from build123d import *

# Parameters (mm, degrees)
SKETCH5_R           = 14
SKETCH5_R_2         = 4
BOSS_EXTRUDE3_DEPTH = 12.5
BOSS_EXTRUDE4_DEPTH = 5


with BuildPart() as part:
    # Sketch5 → Boss-Extrude3 (new body)
    with BuildSketch(Plane(origin=(0, 0, 0), x_dir=(1, 0, 0), z_dir=(0, 1, 0))):
        with Locations(Location((0, 0, 0), (0, 0, 270))):
            Circle(SKETCH5_R)
        with Locations(Location((0, 0, 0), (0, 0, 270))):
            Circle(SKETCH5_R_2, mode=Mode.SUBTRACT)
    extrude(amount=BOSS_EXTRUDE3_DEPTH)

    # Sketch6 → Boss-Extrude4 (add)
    with BuildSketch(Plane(origin=(0, 12.5, 0), x_dir=(1, 0, 0), z_dir=(0, 1, 0))):
        with BuildLine():
            ThreePointArc((0, 14), (-12.934313455, -5.357568053), (9.899494937, -9.899494937))
            ThreePointArc((9.899494937, -9.899494937), (9.899494937, -7.071067812), (7.071067812, -7.071067812))
            ThreePointArc((7.071067812, -7.071067812), (-9.238795325, -3.826834324), (0, 10))
            ThreePointArc((0, 10), (2, 12), (0, 14))
        make_face()
    extrude(amount=BOSS_EXTRUDE4_DEPTH)


solid = part.part
Design review of the part built by this model. Coordinates are the model's own, in mm. A direction names the side the tool comes from. Give positions to 0.01 mm unless a question says otherwise; leave off trailing zeros. Write each loop counter-clockwise with the first axis right and the second up, starting at its lowest first coordinate (ties: lowest second). Pieces come first, ordered by that corner, then holes. Notation, with made-up numbers: M 16.25,-4 L 72.25,-4 A23 ccw 72.25,26 Z; hole C -21,68.5 d9. An arc over 180 degrees is marked long. Return JSON: item names as keys, results as strings. Group by question number.
Item 1: Take a section at B-B (x = -3). Give the boundary of the cut face in (y, z).
Item 2: Tool access review of faces 5 (the flat face through (-3, 0, 3)), 6 (the cylindrical face through (9.93, 14.96, 7.1)): name each direction out of +Z, -Z, +X, -X, +Y, -Y from which nothing blocks a thin tool from reaching the whole face with its end or side.
Item 3: Take a section at C-C (y = 6.5). Give the boundary of the cut face in (x, z), plus the area to 3 significant figures.
Item 4: Wall thickness on line 1 along X through (y, z) = (4.5, 0); line 2 along Y through (x, z) = (7.5, -9); line 3 along X through (y, z) = (13.85, 0): over which ranges is each line inside the solid? List them lowest first.
Item 5: The part is to be moulded in two halves that separate along X. For faces 1 (the cylindrical face through (-9.13, 14.96, 4.08)), 2 (the flat face through (-9, 17.5, 5)), 3 (the cylindrical face through (2, 15, -12)), 4 (the cylindrical face through (-3.905, 6.162, -0.867)), say which applies: pulls with the +X half, pulls with the -X half, needs draft (parallel to the pull), parting line crosses it, or undercut.
Item 6: Take a section at A-A (z = 0). Give the boundary of the cut face in (x, y), plus the area to 3 significant figures.
Item 7: Clearance check with flat-ended pins moving along their axes: pin 1 Ø12 at (x, z) = (0.5, -3) entering from +Y; pin 2 Ø3 at (x, y) = (-4.5, 6.5) entering from -Z; pin 3 Ø1 at (x, y) = (10, 14.5) entering from +Z. State where each tip first meets the part, or that it passes through.
Item 8: Take a section at D-D (z = -6.25). Give the boundary of the cut face in (x, y).
Return value:
{
 "1": {"outline": "M 0,-13.67 L 17.5,-13.67 L 17.5,-9.54 L 12.5,-9.54 L 12.5,-2.65 L 0,-2.65 Z; M 0,2.65 L 12.5,2.65 L 12.5,9.54 L 17.5,9.54 L 17.5,13.67 L 0,13.67 Z"},
 "2": {"face 5": "+Z, -Z, +X, -X, -Y", "face 6": "+Y"},
 "3": {"outline": "C 0,0 d28; hole C 0,0 d8", "area": "565 mm2"},
 "4": {"line 1": "x = -14 to -4, 4 to 14", "line 2": "y = 0 to 12.5", "line 3": "x = -14 to -10"},
 "5": {"face 1": "undercut", "face 2": "needs draft", "face 3": "pulls with the +X half", "face 4": "undercut"},
 "6": {"outline": "M -14,0 L -4,0 L -4,12.5 L -10,12.5 L -10,17.5 L -14,17.5 Z; M 4,0 L 14,0 L 14,12.5 L 4,12.5 Z", "area": "270 mm2"},
 "7": {"pin 1": "stops at y = 12.5", "pin 2": "stops at z = -13.67", "pin 3": "stops at z = 10.28"},
 "8": {"outline": "M -12.53,0 L 12.53,0 L 12.53,12.5 L -7.81,12.5 L -7.81,17.5 L -12.53,17.5 Z"}
}
